from build123d import *

# Parameters (mm, degrees)
BOSS_EXTRUDE1_DEPTH      = 4.5
BOSS_EXTRUDE1_DEPTH_BACK = 4.5
SKETCH3_R                = 1.5


# Read off the part's stored shape, not the designer's step: Cut-Extrude1
with BuildPart() as part:
    # Sketch3 → Boss-Extrude1 (new, two sides: drawn at the far end of the back side and taken through both)
    with BuildSketch(Plane.XY.offset(-BOSS_EXTRUDE1_DEPTH_BACK)):
        Polygon((0, 3.464101615), (-3, 1.732050808), (-3, -1.732050808), (0, -3.464101615), (3, -1.732050808), (3, 1.732050808), align=None)
        Circle(SKETCH3_R, mode=Mode.SUBTRACT)
    extrude(amount=BOSS_EXTRUDE1_DEPTH + BOSS_EXTRUDE1_DEPTH_BACK)

    # Cut-Extrude1 outline → Cut-Extrude1 (revolve, cut)
    with BuildSketch(Plane.XZ):
        Polygon((3.464101616, 4.5), (3, 4.5), (3.464101609, 4.232050811), align=None)
    cut_extrude1 = revolve(axis=Axis((0, 0, 0), (0, 0, 1)), mode=Mode.SUBTRACT)

    # Mirror1: Cut-Extrude1 across plane
    add(cut_extrude1.mirror(Plane.XY), mode=Mode.SUBTRACT)


solid = part.part
Input: part model. Units: mm. Frame: model coordinates. Give positions to 0.01 mm unless a question says otherwise; leave off trailing zeros. Loops run counter-clockwise (first coordinate to the right, second up) from the corner with the lowest first, then second, coordinate; pieces in that order, holes last. Notation, with made-up numbers: (31.25, 80) -> (79.25, 80) arc R19 cw to (79.25, 104) -> close; hole circle Ø2 at (-23, 23). An arc over 180 degrees is marked (long way). Answer as a JSON object with one key per item and string values. Group by question number.
Item 1: Line query: probe 1 along Y at (x, z) = (0.9, -1.5); probe 2 along Y at (x, z) = (-0.45, -3.5); probe 3 along X at (y, z) = (1, -0.75). Output: solid intervals per line, ascending.
Item 2: Cut plane A-A, the plane z = -1.5. Return the cut outline in (x, y), and give its area (3 significant figures).
Item 3: Pull-direction query (X, two-part tool) for faces 1 (the cylindrical face through (-1.5, 0.07, -0.06)), 2 (the conical face through (-2.744, -1.575, 4.405)), 3 (the conical face through (0.008, 3.164, 4.405)); classes: released by +X, released by -X, zero draft, split by the parting line, or undercut.
Item 4: Pin query (flat end, axial travel): P1, Ø1, axis at x = -2, z = 0.5, coming from the +Y side; P2, Ø1.8, axis at x = 0, y = 0, coming from the -Z side; P3, Ø1, axis at y = -3, z = 1, coming from the -X side; P4, Ø2, axis at x = -2, z = 1, coming from the -Y side. Return the tip coordinate at first contact, or that it passes through.
Checks:
{
 "1": {"probe 1": "y = -2.94 to -1.2, 1.2 to 2.94", "probe 2": "y = -3.2 to -1.43, 1.43 to 3.2", "probe 3": "x = -3 to -1.12, 1.12 to 3"},
 "2": {"outline": "(-3, -1.73) -> (0, -3.46) -> (3, -1.73) -> (3, 1.73) -> (0, 3.46) -> (-3, 1.73) -> close; hole circle Ø3 at (0, 0)", "area": "24.1 mm²"},
 "3": {"face 1": "undercut", "face 2": "released by -X", "face 3": "split by the parting line"},
 "4": {"P1": "stops at y = 2.6", "P2": "passes through", "P3": "stops at x = -1.67", "P4": "stops at y = -2.89"}
}
